Verification items for the finished model (mm, model axes). A direction names the side the tool comes from. Coordinates: 2 decimals unless noted, no trailing zeros. Loops run counter-clockwise (first coordinate to the right, second up) from the corner with the lowest first, then second, coordinate; pieces in that order, holes last. Notation, with made-up numbers: (0, 56) -> (15, 56) arc R21 ccw to (15, 81) -> close; hole circle Ø5 at (-35, 62). An arc over 180 degrees is marked (long way). Write item = value, one per line.
```python
from build123d import *

# Parameters (mm, degrees)
F3_R        = 16
F4_DEPTH    = 60
F2_R        = 6
F0_R        = 13.5
F4_FACE_R   = 16
F4_FACE_R_2 = 6
F6_DEPTH    = 2


with BuildPart() as f4:
    # F3 (on Top) → F4 (new body)
    with BuildSketch(Plane.XY):
        Circle(F3_R)
    extrude(amount=F4_DEPTH)

    # F2 (on offset) → F5 section 0
    with BuildSketch(Plane.XY.offset(60)):
        Circle(F2_R)
    # F0 (on Top) → F5 section 1
    with BuildSketch(Plane.XY):
        Circle(F0_R)
    loft(mode=Mode.SUBTRACT)

    # F2 (on offset) + F4_face (on face) → F6 (join)
    with BuildSketch(Plane.XY.offset(60)):
        Circle(F2_R)
    with BuildSketch(Plane.XY.offset(60)):
        Circle(F4_FACE_R)
        Circle(F4_FACE_R_2, mode=Mode.SUBTRACT)
    extrude(amount=F6_DEPTH)


solid = f4.part
```
1) Sectioned sample at B-B, the plane z = 48. Record the cut outline in (x, y).
Ans:
outline = circle Ø32 at (0, 0); hole circle Ø15 at (0, 0)
2) Sectioned sample at C-C, the plane z = 25.5. Record the cut outline in (x, y) (1 decimal).
Ans:
outline = circle Ø32 at (0, 0); hole circle Ø20.6 at (0, 0)
3) Sectioned sample at D-D, the plane x = 14.5. Record the cut outline in (y, z).
Ans:
outline = (-6.76, 0) -> (6.76, 0) -> (6.76, 62) -> (-6.76, 62) -> close
4) Sectioned sample at A-A, the plane x = 0. Record the cut outline in (y, z).
Ans:
outline = (-16, 0) -> (-13.5, 0) -> (-6, 60) -> (6, 60) -> (13.5, 0) -> (16, 0) -> (16, 62) -> (-16, 62) -> close
5) Depth check by flat-ended pin: pin 1 Ø4 at (y, z) = (7.5, 35.5) entering from -X (3 decimals); pin 2 Ø9.5 at (x, y) = (0.5, 0) entering from -Z; pin 3 Ø8 at (y, z) = (-6, 28.5) entering from -X. Enter the tip coordinate at first touch or a pass-through.
Ans:
pin_1 = -15.025
pin_2 = 60
pin_3 = -15.87
6) Material ranges on line 1 (Z direction, x = -1, y = -3); line 2 (Y direction, x = 1.5, z = 46); line 3 (Y direction, x = -1.5, z = 3), recorded low to high.
Ans:
line_1 = 60 to 62
line_2 = -15.93 to -7.6, 7.6 to 15.93
line_3 = -15.93 to -13.04, 13.04 to 15.93
7) Tool access check on faces 4 (the face through (-7, -12, 0)), 5 (the face through (0, 0, 60)). Record the directions out of +Z, -Z, +X, -X, +Y, -Y that give a thin tool (end or side, any length) a straight path to the whole face; none if there is none.
Ans:
face_4 = -Z, +X, -X, +Y, -Y
face_5 = -Z
8) Release check for a two-part mould opening along Y. For faces 1 (the face through (-3.47, -15.62, 30.57)), 2 (the face through (0, 0, 62)), 3 (the face through (9.35, 2.94, 29.58)) record: pulls with the +Y half, pulls with the -Y half, needs draft (parallel to the pull), parting line crosses it, or undercut.
Ans:
face_1 = parting line crosses it
face_2 = needs draft
face_3 = undercut
